Read the model definition and answer for the solid it produces. Units are mm, in the model's axes. A direction names the side the tool comes from. Coordinates: 2 decimals unless noted, no trailing zeros. Order: outer loops, then holes, each group sorted by start corner. A loop starts at its lowest first (then second) coordinate and runs counter-clockwise, first axis right, second up.
```python
from build123d import *

# Parameters (mm, degrees)
SZKIC1_R                        = 3
DODANIE_WYCI_GNI_CIE1_DEPTH     = 13
SZKIC2_R                        = 3.83
DODANIE_WYCI_GNI_CIE2_DEPTH     = 9
GWINT1_PITCH                    = 1.25
SZKIC6_R                        = 6
DODANIE_WYCI_GNI_CIE3_DEPTH     = 2
SZKIC8_W                        = 15.88
SZKIC8_H                        = 21.21
DODANIE_WYCI_GNI_CIE4_DEPTH     = 14
ZAOKR_GLENIE1_R                 = 2
WYTNIJ_WYCI_GNI_CIE1_DEPTH      = 9
DODANIE_WYCI_GNI_CIE6_OUTLINE_W = 1
DODANIE_WYCI_GNI_CIE6_OUTLINE_H = 2
DODANIE_WYCI_GNI_CIE6_ANGLE     = 180
DODANIE_WYCI_GNI_CIE7_START     = 24
DODANIE_WYCI_GNI_CIE7_DEPTH     = 1
WYTNIJ_WYCI_GNI_CIE2_START      = -13
SZKIC11_R                       = 50
WYTNIJ_WYCI_GNI_CIE2_DEPTH      = 28.69554901


# Read off the part's stored shape, not the designer's step: Dodanie-wyciągnięcie6
with BuildPart() as part:
    # Szkic1 → Dodanie-wyciągnięcie1 (new body)
    with BuildSketch(Plane.XY):
        with Locations(Location((0, 0, 0), (0, 0, 180))):
            Circle(SZKIC1_R)
    extrude(amount=DODANIE_WYCI_GNI_CIE1_DEPTH)

    # Szkic2 → Dodanie-wyciągnięcie2 (add)
    with BuildSketch(Plane.XY.offset(13)):
        Circle(SZKIC2_R)
    extrude(amount=DODANIE_WYCI_GNI_CIE2_DEPTH)

    # Gwint1: the profile of Profil gwintu1 profile screwed along a right-hand helix of 8 turns, 8 arcs to a turn; built about Z, then put on its axis
    gwint1_z = Axis((0, 0, 0), (0, 0, 1))
    gwint1_corners = [(3.8297, 0, -0.000173205), (4.506582344, 0, 0.390624998), (4.506582344, 0, 0.546874998), (3.8297, 0, 0.937673202)]
    with BuildLine(mode=Mode.PRIVATE) as gwint1_profile:
        Line(gwint1_corners[0], gwint1_corners[1])
        Line(gwint1_corners[1], gwint1_corners[2])
        Line(gwint1_corners[2], gwint1_corners[3])
        Line(gwint1_corners[3], gwint1_corners[0])
    gwint1_cap = Face(gwint1_profile.wire())
    gwint1_turn_angles = [0, 22.5, 45, 67.5, 90, 112.5, 135, 157.5, 180, 202.5, 225, 247.5, 270, 292.5, 315, 337.5, 360]
    gwint1_turn_weights = [1, 0.9238795325112867, 1, 0.9238795325112867, 1, 0.9238795325112867, 1, 0.9238795325112867, 1, 0.9238795325112867, 1, 0.9238795325112867, 1, 0.9238795325112867, 1, 0.9238795325112867, 1]
    gwint1_turn_rails = [Edge.make_bspline([Vector(p[0], p[1], 0).rotate(gwint1_z, gwint1_turn_angles[k]) / gwint1_turn_weights[k] + Vector(0, 0, p[2] + GWINT1_PITCH * gwint1_turn_angles[k] / 360) for k in range(17)], [0, 0, 0, 1, 1, 2, 2, 3, 3, 4, 4, 5, 5, 6, 6, 7, 7, 8, 8, 8], 2, gwint1_turn_weights) for p in gwint1_corners]
    gwint1_turn_sides = [Face.make_surface_from_curves(gwint1_turn_rails[p[0]], gwint1_turn_rails[p[1]]) for p in [(0, 1), (1, 2), (2, 3), (3, 0)]]
    gwint1 = Plane(origin=(0, 0, 13), x_dir=(1, 0, 0), z_dir=(0, 0, 1)) * Solid(Shell([*[p.moved(Location((0, 0, GWINT1_PITCH * i))) for i in range(8) for p in gwint1_turn_sides], gwint1_cap, gwint1_cap.rotate(gwint1_z, 2880).moved(Location((0, 0, GWINT1_PITCH * 2880 / 360)))]))
    add(gwint1)

    # Szkic6 → Dodanie-wyciągnięcie3 (add)
    with BuildSketch(Plane.XY.offset(22)):
        Circle(SZKIC6_R)
    extrude(amount=DODANIE_WYCI_GNI_CIE3_DEPTH)

    # Szkic8 → Dodanie-wyciągnięcie4 (add)
    with BuildSketch(Plane.XY.offset(24)):
        with Locations((0, -1.605)):
            Rectangle(SZKIC8_W, SZKIC8_H)
    extrude(amount=DODANIE_WYCI_GNI_CIE4_DEPTH)

    # Zaokrąglenie1
    zaokr_glenie1_edges = [part.edges().sort_by_distance(p)[0] for p in [
        (-7.94, -1.605, 24),
        (-7.94, 9, 31),
        (0, -12.21, 24),
        (-7.94, -12.21, 31),
        (7.94, -1.605, 24),
        (7.94, -12.21, 31),
        (0, 9, 24),
        (7.94, 9, 31),
    ]]
    fillet(zaokr_glenie1_edges, radius=ZAOKR_GLENIE1_R)

    # Szkic9 → Wytnij-wyciągnięcie1 (cut)
    with BuildSketch(Plane(origin=(0, 0, 0), x_dir=(-1, 0, 0), z_dir=(0, 0, -1))):
        Polygon((-1.596370884, -2.54), (1.596370884, -2.54), (8.034501067, -6.687500384), (-7.848069709, -6.190255995), align=None)
    extrude(amount=-WYTNIJ_WYCI_GNI_CIE1_DEPTH, mode=Mode.SUBTRACT)

    # Dodanie-wyciągnięcie6 outline → Dodanie-wyciągnięcie6 (revolve)
    with BuildSketch(Plane.YZ.offset(7.94)):
        with Locations((0.5, 25)):
            Rectangle(DODANIE_WYCI_GNI_CIE6_OUTLINE_W, DODANIE_WYCI_GNI_CIE6_OUTLINE_H)
    revolve(axis=Axis((7.94, 0, 0), (0, 0, 1)), revolution_arc=DODANIE_WYCI_GNI_CIE6_ANGLE)

    # Szkic10<2> → Dodanie-wyciągnięcie7 (add)
    with BuildSketch(Plane.XY.offset(DODANIE_WYCI_GNI_CIE7_START)):
        with BuildLine():
            Line((7.94, 0), (7.94, 1))
            ThreePointArc((7.94, 1), (6.94, 0), (7.94, -1))
            Line((7.94, -1), (7.94, 0))
        make_face()
    extrude(amount=-DODANIE_WYCI_GNI_CIE7_DEPTH)

    # Szkic11 → Wytnij-wyciągnięcie2 (cut, through all)
    with BuildSketch(Plane(origin=(0, 0, 0), x_dir=(-1, 0, 0), z_dir=(0, 0, -1)).offset(WYTNIJ_WYCI_GNI_CIE2_START)):
        Circle(SZKIC11_R)
    extrude(amount=-WYTNIJ_WYCI_GNI_CIE2_DEPTH, mode=Mode.SUBTRACT)


with BuildPart() as wytnij_wyci_gni_cie2_kept_piece:
    # of the separate pieces the step leaves, the one the design keeps (wytnij_wyci_gni_cie2_pieces_kept)
    add(part.part.solids().sort_by_distance((-3, 0, 0))[0])


solid = wytnij_wyci_gni_cie2_kept_piece.part
```
1) A cutting plane is placed at A-A, the plane x = 0. Determine the outline of the cut face in (y, z).
A:
outline: (-3, 9) - (-2.54, 9) - (-2.54, 0) - (3, 0) - (3, 13) - (-3, 13) - close
2) Flat-ended cylindrical pins translate along their axes: pin 1 Ø1 at (x, z) = (0.5, 2.5) entering from -Y; pin 2 Ø1.5 at (y, z) = (-2, 2) entering from -X. Find the tip coordinate at first contact, or state that the pin passes through.
A:
pin 1: stops at y = -2.54
pin 2: stops at x = -2.73
3) A cutting plane is placed at D-D, the plane z = 10.25. Determine the outline of the cut face in (x, y).
A:
outline: circle Ø6 at (0, 0)
4) Straight lines are drawn through the part: line 1 (X direction, y = -0.1, z = 6.25); line 2 (X direction, y = 2.25, z = 2.75); line 3 (Y direction, x = -1.95, z = 1.5). For each, find the intervals that lie inside material, in ascending order.
A:
line 1: x = -3 to 3
line 2: x = -1.98 to 1.98
line 3: y = -2.28 to 2.28
5) A cutting plane is placed at B-B, the plane z = 7. Determine the outline of the cut face in (x, y), and give its area (3 significant figures).
A:
outline: (-1.6, -2.54) - (1.6, -2.54) arc R3 ccw (long way) to start
area: 27.3 mm2
6) Which of the six approach directions +Z, -Z, +X, -X, +Y, -Y give full straight-line access (tool end or side, diameter ignored) to faces 1 (the flat face through (0, 0, 0)), 2 (the flat face through (0, -2.54, 4))?
A:
face 1: -Z, +X, -X, +Y, -Y
face 2: -Z, +X, -X, -Y
7) A cutting plane is placed at C-C, the plane y = -2.2. Determine the outline of the cut face in (x, z).
A:
outline: (-2.04, 0) - (2.04, 0) - (2.04, 13) - (-2.04, 13) - close
